Input: part model. Units: mm. Frame: model coordinates. A direction names the side the tool comes from. Coordinates: 2 decimals unless noted, no trailing zeros. Loops run counter-clockwise (first coordinate to the right, second up) from the corner with the lowest first, then second, coordinate; pieces in that order, holes last. Notation, with made-up numbers: (14, 86.25) - (19, 86.25) arc R20 cw to (19, 108.25) - close; hole circle Ø8 at (25.25, 5.5). An arc over 180 degrees is marked (long way). Use a Markdown table: item, result. Add a question column.
1. Section query A-A on y = -20.4. Return the cut outline in (x, z), then the cut area to 3 significant figures.
2. Section query D-D on y = -17.75. Return the cut outline in (x, z), then the cut area to 3 significant figures.
3. Section query B-B on x = -7.91. Return the cut outline in (y, z).
4. Draft query along Y for faces 6 (the face through (0.503, -13.457, -27.485)), 7 (the face through (-0.4, -7.8, -25.9)), 8 (the face through (-2, -12, -19.45)), 9 (the face through (10.16, -1, -7)). Return one class per face: released by +Y, released by -Y, zero draft, split by the parting line, or undercut.
5. Access query for faces 1 (the face through (-8.05, -19.31, 20.77)), 2 (the face through (-5, -12, 19.55)), 3 (the face through (7.16, -12.55, -18.18)), 4 (the face through (1, -12, -24.95)), 5 (the face through (10.16, -24, -7)). Directions: +Z, -Z, +X, -X, +Y, -Y. A direction counts if a zero-diameter tool reaches every point of the face in a straight line with its end or side. Return the directions, or none.
6. Ray query, L1, parallel to Y at x = -7.91, z = 20.3; L2, parallel to X at y = -12.45, z = -28.6; L3, parallel to Y at x = 3, z = -16. Return the intervals inside material, ascending. Write a range as [from, to].
7. Contact query for flat-ended pins moving along their axis: P1, Ø1.5, axis at x = 1.5, y = -10, coming from the +Z side; P2, Ø3, axis at x = 7, y = -12.5, coming from the +Z side; P3, Ø1.8, axis at x = -7.91, y = -4.5, coming from the +Z side. Output: stop coordinate, or through.
8. Section query C-C on z = -6.5. Return the cut outline in (x, y).
```python
from build123d import *

# Parameters (mm, degrees)
F1_DEPTH  = 24.9
F2_W      = 19.9
F2_H      = 36.5
F3_DEPTH  = 25.4
F4_W      = 24.9
F4_H      = 5
F4_H_2    = 7.5
F5_DEPTH  = 2.5
F7_DEPTH  = 2.5
F8_R      = 1.1
F9_DEPTH  = 25.4
F10_R     = 4.7625
F11_DEPTH = 8
F12_R     = 1.016
F13_DEPTH = 5
F14_W     = 2.5
F14_H     = 7.5
F14_H_2   = 5
F15_DEPTH = 25.4
F16_W     = 24.9
F16_H     = 7.5
F17_DEPTH = 2.5


with BuildPart() as f1:
    # F0 (on Front) → F1 (new body)
    with BuildSketch(Plane.XZ):
        Polygon((10.16, 0), (0, 21.95), (-10.16, 21.95), (-10.16, -21.95), (10.16, -21.95), align=None)
    extrude(amount=F1_DEPTH)

    # F2 (on face) → F3 (cut)
    with BuildSketch(Plane(origin=(-10.16, 0, 0), x_dir=(0, -1, 0), z_dir=(-1, 0, 0))):
        with Locations((12.45, 1.3)):
            Rectangle(F2_W, F2_H)
    extrude(amount=-F3_DEPTH, mode=Mode.SUBTRACT)

    # F4 (on face) → F5 (join)
    with BuildSketch(Plane(origin=(-10.16, 0, 0), x_dir=(0, -1, 0), z_dir=(-1, 0, 0))):
        with Locations((12.45, 19.45)):
            Rectangle(F4_W, F4_H)
        with Locations((12.45, -18.2)):
            Rectangle(F4_W, F4_H_2)
    extrude(amount=F5_DEPTH)

    # F6 (on face) → F7 (cut)
    with BuildSketch(Plane.XY.offset(-16.95)):
        with BuildLine():
            Line((4.36, -6.370526), (4.36, -2.5))
            Line((4.36, -2.5), (-10.16, -2.5))
            Line((-10.16, -2.5), (-10.16, -22.4))
            Line((-10.16, -22.4), (4.36, -22.4))
            Line((4.36, -22.4), (4.36, -18.529474))
            ThreePointArc((4.36, -18.529474), (7.16, -12.45), (4.36, -6.370526))
        make_face()
    extrude(amount=-F7_DEPTH, mode=Mode.SUBTRACT)

    # F8 (on face) → F9 (cut)
    with BuildSketch(Plane.XY.offset(21.95)):
        with Locations((-7.91, -4.5)):
            Circle(F8_R)
        with Locations((-7.91, -20.4)):
            Circle(F8_R)
    extrude(amount=-F9_DEPTH, mode=Mode.SUBTRACT)

    # F10 (on face) → F11 (join)
    with BuildSketch(Plane(origin=(0, 0, -21.95), x_dir=(1, 0, 0), z_dir=(0, 0, -1))):
        with Locations((0.635, 12.45)):
            Circle(F10_R)
    extrude(amount=F11_DEPTH)

    # F12 (on face) → F13 (cut)
    with BuildSketch(Plane(origin=(0, 0, -29.95), x_dir=(1, 0, 0), z_dir=(0, 0, -1))):
        with Locations((0.635, 12.45)):
            Circle(F12_R)
    extrude(amount=-F13_DEPTH, mode=Mode.SUBTRACT)

    # F14 (on face) → F15 (cut)
    with BuildSketch(Plane.XZ.offset(24.9)):
        with Locations((-11.41, -18.2)):
            Rectangle(F14_W, F14_H)
        with Locations((-11.41, 19.45)):
            Rectangle(F14_W, F14_H_2)
    extrude(amount=-F15_DEPTH, mode=Mode.SUBTRACT)

    # F16 (on face) → F17 (join)
    with BuildSketch(Plane.YZ.offset(10.16)):
        with Locations((-12.45, -18.2)):
            Rectangle(F16_W, F16_H)
    extrude(amount=F17_DEPTH)


solid = f1.part
```
Resolved:
| question | item | result |
|---|---|---|
| 1 | outline | (-10.16, -21.95) - (12.66, -21.95) - (12.66, -14.45) - (10.16, -14.45) - (10.16, -16.95) - (4.36, -16.95) - (4.36, -19.45) - (-10.16, -19.45) - close; (-10.16, 19.55) - (-9.01, 19.55) - (-9.01, 21.95) - (-10.16, 21.95) - close; (-6.81, 19.55) - (1.11, 19.55) - (0, 21.95) - (-6.81, 21.95) - close |
| 1 | area | 104 mm² |
| 2 | outline | (-10.16, -21.95) - (12.66, -21.95) - (12.66, -14.45) - (10.16, -14.45) - (10.16, -16.95) - (5.15, -16.95) - (5.15, -19.45) - (-10.16, -19.45) - close; (-10.16, 19.55) - (1.11, 19.55) - (0, 21.95) - (-10.16, 21.95) - close |
| 2 | area | 108 mm² |
| 3 | outline | (-24.9, -21.95) - (0, -21.95) - (0, 21.95) - (-3.4, 21.95) - (-3.4, 19.55) - (-2.5, 19.55) - (-2.5, -19.45) - (-22.4, -19.45) - (-22.4, 19.55) - (-21.5, 19.55) - (-21.5, 21.95) - (-24.9, 21.95) - close; (-19.3, 19.55) - (-5.6, 19.55) - (-5.6, 21.95) - (-19.3, 21.95) - close |
| 4 | face 6 | undercut |
| 4 | face 7 | split by the parting line |
| 4 | face 8 | undercut |
| 4 | face 9 | zero draft |
| 5 | face 1 | +Z |
| 5 | face 2 | +X, -X |
| 5 | face 3 | +Z, -X |
| 5 | face 4 | -Z |
| 5 | face 5 | +Z, +X, +Y, -Y |
| 6 | L1 | [-24.9, -21.5], [-19.3, -5.6], [-3.4, 0] |
| 6 | L2 | [-4.13, -0.38], [1.65, 5.4] |
| 6 | L3 | [-24.9, -22.4], [-2.5, 0] |
| 7 | P1 | z = 20.33 |
| 7 | P2 | z = -16.95 |
| 7 | P3 | z = -19.45 |
| 8 | outline | (-10.16, -24.9) - (10.16, -24.9) - (10.16, -22.4) - (-10.16, -22.4) - close; (-10.16, -2.5) - (10.16, -2.5) - (10.16, 0) - (-10.16, 0) - close |
